```python
from build123d import *

# Parameters (mm, degrees)
SKETCH_1_W                       = 320
SKETCH_1_H                       = 10
EXTRUDE_1_DEPTH                  = 10
SKETCH_2_R                       = 4
CUT_EXTRUDE_1_DEPTH              = 1270
CUT_EXTRUDE_2_DEPTH              = 1270
FILLET_1_R                       = 1
PATTERN_CIRCULAR_2_COUNT         = 4
FILLET_1_OF_PATTERN_CIRCULAR_2_R = 1
CUT_EXTRUDE_4_DEPTH              = 24


with BuildPart() as part:
    # 草图1 → 凸台-拉伸1 (new body)
    with BuildSketch(Plane.XY):
        with Locations((93.481285353, -6.397869645)):
            Rectangle(SKETCH_1_W, SKETCH_1_H)
    extrude_1 = extrude(amount=EXTRUDE_1_DEPTH)

    # 草图2 → 切除-拉伸1 (cut)
    with BuildSketch(Plane(origin=(253.481285353, 0, 0), x_dir=(0, 0, -1), z_dir=(1, 0, 0))):
        with Locations((0, -11.397869645)):
            Circle(SKETCH_2_R)
    cut_extrude_1 = extrude(amount=-CUT_EXTRUDE_1_DEPTH, mode=Mode.SUBTRACT)

    # 草图3 → 切除-拉伸2 (cut)
    with BuildSketch(Plane(origin=(253.481285353, 0, 0), x_dir=(0, 0, -1), z_dir=(1, 0, 0))):
        Polygon((-4, -1.397869645), (0, -1.397869645), (0, -5.397869645), (-3, -5.397869645), (-5.5, -1.897869645), (-4, -1.897869645), align=None)
        Polygon((-10, -7.397869645), (-10, -11.397869645), (-6, -11.397869645), (-6, -8.397869645), (-9.5, -5.897869645), (-9.5, -7.397869645), align=None)
    cut_extrude_2 = extrude(amount=-CUT_EXTRUDE_2_DEPTH, mode=Mode.SUBTRACT)

    # 圆角1
    fillet_1_edges = [part.edges().sort_by_distance(p)[0] for p in [
        (93.481285353, -1.397869645, 10),
    ]]
    fillet(fillet_1_edges, radius=FILLET_1_R)

    # 阵列(圆周)2: 凸台-拉伸1, 切除-拉伸1, 切除-拉伸2 ×4 about axis
    pattern_circular_2_axis = Axis((0, -11.397869645, 0), (1, 0, 0))
    add([extrude_1.rotate(pattern_circular_2_axis, i * 360 / PATTERN_CIRCULAR_2_COUNT) for i in range(1, PATTERN_CIRCULAR_2_COUNT)])
    add([cut_extrude_1.rotate(pattern_circular_2_axis, i * 360 / PATTERN_CIRCULAR_2_COUNT) for i in range(1, PATTERN_CIRCULAR_2_COUNT)], mode=Mode.SUBTRACT)
    add([cut_extrude_2.rotate(pattern_circular_2_axis, i * 360 / PATTERN_CIRCULAR_2_COUNT) for i in range(1, PATTERN_CIRCULAR_2_COUNT)], mode=Mode.SUBTRACT)

    # 圆角1 of 阵列(圆周)2
    fillet_1_of_pattern_circular_2_edges = [part.edges().sort_by_distance(p)[0] for p in [
        (93.481285353, -21.397869645, 10),
        (93.481285353, -21.397869645, -10),
        (93.481285353, -1.397869645, -10),
    ]]
    fillet(fillet_1_of_pattern_circular_2_edges, radius=FILLET_1_OF_PATTERN_CIRCULAR_2_R)

    # 草图5 → 切除-拉伸4 (cut)
    with BuildSketch(Plane.XZ.offset(21.397869645)):
        Polygon((-78.202673037, 13.081723415), (-42.997967066, 30.32515978), (-66.48214009, -10.35062107), align=None)
    extrude(amount=-CUT_EXTRUDE_4_DEPTH, mode=Mode.SUBTRACT)


solid = part.part
```
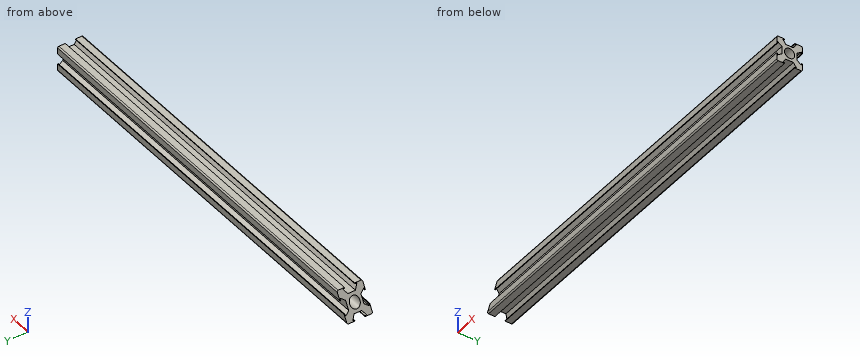
Build history of the part. All positions in model axes, mm. Give positions to 0.01 mm unless a question says otherwise; leave off trailing zeros. Loops run counter-clockwise (first coordinate to the right, second up) from the corner with the lowest first, then second, coordinate; pieces in that order, holes last. Notation, with made-up numbers: (11, -11) -> (40, -11) arc R3 ccw to (40, -6) -> close; hole circle Ø6 at (44, 81). An arc over 180 degrees is marked (long way). One line per question, with ' | ' between items. Start each with the question number.
1) Pin check, flat tips, straight feed: pin 1 (8 mm diameter, centred on y = -8, z = 2, fed in from -X); pin 2 (1.5 mm diameter, centred on x = 160, y = -12.5, fed in from -Z); pin 3 (1.8 mm diameter, centred on x = 65.5, y = -12.5, fed in from +Z). Stop position of each tip, or through.
2) Probe L1, parallel to Z at x = 62.5, y = -16.5; L2, parallel to Y at x = 100, z = 0; L3, parallel to Z at x = 95.5, y = -8.75. List the from-to ranges inside material, lowest first.
3) Cut at A-A (z = 0). Give the cut face in (x, y), plus the area to 3 significant figures.
Return value:
1) pin 1: x = -61.66 | pin 2: z = -6 | pin 3: z = 6
2) L1: -10 to -9.5, -8.94 to 8.94, 9.5 to 10 | L2: -17.4 to -15.4, -7.4 to -5.4 | L3: -6 to -3, 3 to 6
3) outline: (-60.51, -17.4) -> (253.48, -17.4) -> (253.48, -15.4) -> (-60.51, -15.4) -> close; (-60.51, -7.4) -> (253.48, -7.4) -> (253.48, -5.4) -> (-60.51, -5.4) -> close | area: 1,260 mm^2
